Could you check a few things on this model? Use its own coordinates, in mm. A direction names the side the tool comes from. Give positions to 0.01 mm unless a question says otherwise; leave off trailing zeros. Write each loop counter-clockwise with the first axis right and the second up, starting at its lowest first coordinate (ties: lowest second). Pieces come first, ordered by that corner, then holes. Notation, with made-up numbers: (-32, 65.5) - (21, 65.5) arc R17 cw to (21, 91.5) - close; hole circle Ø6 at (29.25, 30.5). An arc over 180 degrees is marked (long way). Answer in a Markdown table with one row per item.
Autodesk Inventor part; units mm, degrees
ref_plane "YZ Plane" through (0, 0, 0) normal (1, 0, 0) x (0, 1, 0)
ref_plane "XZ Plane" through (0, 0, 0) normal (0, 1, 0) x (-1, 0, 0)
ref_plane "XY Plane" through (0, 0, 0) normal (0, 0, 1) x (1, 0, 0)
sketch "スケッチ1" plane through (0, 0, 0) normal (0, 0, 1) x (1, 0, 0)
  circle A0 centre (11, -20) radius 1.25 construction
  circle A1 centre (11, 20) radius 1.25 construction
  circle A2 centre (-11, -20) radius 1.25 construction
  arc A3 (8.5, 20) -> (11, 17.5) centre (11, 20) ccw construction
  line L0 (11, 17.5) -> (12.15, 17.5) construction
  arc A4 (13.15, 16.5) -> (12.15, 17.5) centre (12.15, 16.5) ccw construction
  line L1 (13.15, 16.5) -> (13.15, -16.5) construction
  arc A5 (12.15, -17.5) -> (13.15, -16.5) centre (12.15, -16.5) ccw construction
  line L2 (12.15, -17.5) -> (11, -17.5) construction
  arc A6 (11, -17.5) -> (8.5, -20) centre (11, -20) ccw construction
  line L3 (8.5, -20) -> (8.5, -21.15) construction
  arc A7 (7.5, -22.15) -> (8.5, -21.15) centre (7.5, -21.15) ccw construction
  line L4 (7.5, -22.15) -> (-7.5, -22.15) construction
  arc A8 (-8.5, -21.15) -> (-7.5, -22.15) centre (-7.5, -21.15) ccw construction
  line L5 (-8.5, -21.15) -> (-8.5, -20) construction
  arc A9 (-8.5, -20) -> (-11, -17.5) centre (-11, -20) ccw construction
  line L6 (-11, -17.5) -> (-14, -17.5) construction
  line L7 (8.5, 23) -> (8.5, 20) construction
  line L8 (-14.25, -17.75) -> (-14.25, -21.25) construction
  line L9 (-14.25, -21.25) -> (-12.25, -23.25)
  line L10 (-12.25, -23.25) -> (12.25, -23.25)
  line L11 (12.25, -23.25) -> (14.25, -21.25)
  line L12 (14.25, -21.25) -> (14.25, 21.25) construction
  line L13 (14.25, 21.25) -> (12.25, 23.25)
  line L14 (12.25, 23.25) -> (8.75, 23.25) construction
  line L15 (16.75, 15.618) -> (22.25, 15.618)
  line L16 (41.3, 21.118) -> (41.3, -2.882)
  line L17 (19.75, -0.382) -> (16.75, -0.382)
  arc A10 (41.3, 21.118) -> (35.8184, 22.8038) centre (38.3, 21.118) ccw
  arc A11 (39.5165, -5.6243) -> (41.3, -2.882) centre (38.3, -2.882) ccw
  circle A12 centre (38.3, 21.118) radius 1.25 construction
  circle A13 centre (38.3, -2.882) radius 1.25 construction
  line L18 (14.25, 21.25) -> (14.25, 18.118)
  line L19 (14.25, -2.882) -> (14.25, -21.25)
  arc A14 (14.25, 18.118) -> (16.75, 15.618) centre (16.75, 18.118) ccw
  arc A15 (16.75, -0.382) -> (14.25, -2.882) centre (16.75, -2.882) ccw
  line L20 (72.306, -6.882) -> (-28.676, -6.882) construction
  circle A16 centre (1.21, -13.01) radius 8.7 construction
  circle A17 centre (1.21, -13.01) radius 8.95
  arc A18 (22.25, 15.618) -> (35.8184, 22.8038) centre (22.25, 32.0211) ccw
  line L21 (22.25, 32.0211) -> (22.25, -5.382) construction
  line L22 (22.25, -2.882) -> (22.25, -5.882)
  line L23 (24.75, -8.382) -> (33.3, -8.382)
  line L24 (33.3, -8.382) -> (39.5165, -5.6243)
  arc A19 (22.25, -2.882) -> (19.75, -0.382) centre (19.75, -2.882) ccw
  arc A20 (22.25, -5.882) -> (24.75, -8.382) centre (24.75, -5.882) ccw
  circle A21 centre (0, 12) radius 1.25 construction
  line L25 (12.25, 23.25) -> (8.5, 23.25)
  line L26 (8.5, 23.25) -> (-2.0647, 20.76)
  arc A22 (-2.0647, 20.76) -> (-8.234, 15.6334) centre (0, 12) ccw
  line L27 (0, 0) -> (0, -31.805) construction
  line L28 (-12.15, -17.5) -> (-14.25, -17.5) construction
  line L29 (8.5, 23.25) -> (8.5, 21.15) construction
  line L30 (8.75, 23.25) -> (8.5, 23)
  line L31 (-14, -17.5) -> (-14.25, -17.75) construction
  line L32 (-14.25, 0) -> (-14.25, -2) construction
  line L33 (-14.25, -2) -> (-16.25, -2)
  line L34 (-16.25, -2) -> (-16.25, -5)
  line L35 (-16.25, -5) -> (-14.25, -5)
  line L36 (-14.25, -5) -> (-14.25, -7) construction
  line L37 (-14.25, 0) -> (-14.25, 2)
  line L38 (-14.25, 2) -> (-8.234, 15.6334)
  arc A23 (-14.25, -2) -> (-14.25, 0) centre (-14.25, -1) ccw
  arc A24 (-14.25, -7) -> (-14.25, -5) centre (-14.25, -6) ccw
  line L39 (-14.25, -7) -> (-14.25, -21.25)
  point P0 (11, 20)
  point P1 (11, -20)
  point P2 (-11, -20)
  point P3 (14.25, 15.618)
  point P4 (23.6679, 15.618)
  point P5 (23.161, -0.382)
  point P6 (14.25, -0.382)
  point P7 (22.25, -0.382)
  dimension "d0" = 3
  dimension "d1" = 2.5
  dimension "d2" = 6.5
  dimension "d3" = 0.25
  dimension "d7" = 16
  dimension "d8" = 8
  dimension "d16" = 8
  dimension "d17" = 5
  dimension "d26" = 9
  dimension "d34" = 1
  dimension "d35" = 3
  dimension "d36" = 2
  dimension "d37" = 10
  dimension "d38" = 2
extrude "押し出し1" add sketch "スケッチ1" along normal blind 2
sketch "スケッチ2" plane through (0, 0, 2) normal (0, 0, 1) x (1, 0, 0)
  point P0 (0, 0)
  point P1 (38.3, 21.118)
  point P2 (38.3, -2.882)
  point P3 (-11, 20)
  point P4 (11, 20)
  point P5 (11, -20)
  point P6 (-11, -20)
hole "穴2" at (38.3, 21.118, 2) at (38.3, -2.882, 2) at (-11, 20, 2) at (11, 20, 2) at (11, -20, 2) at (-11, -20, 2) direction (0, 0, -1) diameter 2.5 end through all countersink diameter 5 countersink angle 90
hole "穴3" at (0, 12, 0) direction (0, 0, 1) diameter 3 end through all
chamfer "面取り1" distance 0.25 angle 45 2 edges at (-16.25, -2, 1) (-16.25, -5, 1)
properties part number "COXA_YAW_ROLL_ADPT_TOP_BASE"
1) Imagine slicing it at A-A (y = -13.01). List the corners of the cut face in (x, z) for me.
Check values:
| item | result |
|---|---|
| outline | (-14.25, 0) - (-7.74, 0) - (-7.74, 2) - (-14.25, 2) - close; (10.16, 0) - (14.25, 0) - (14.25, 2) - (10.16, 2) - close |
2) Imagine slicing it at B-B (x = -11). List the corners of the cut face in (y, z) for me.
Check values:
| item | result |
|---|---|
| outline | (-23.25, 0) - (-21.25, 0) - (-21.25, 0.75) - (-22.5, 2) - (-23.25, 2) - close; (-18.75, 0) - (9.37, 0) - (9.37, 2) - (-17.5, 2) - (-18.75, 0.75) - close |
3) We'd pull the mould along Y, two halves only. Please class faces 1 (the face through (39.52, -2.61, 0.37)), 2 (the face through (-11.284, 8.721, 0.986)), 3 (the face through (14.25, 20, 1)): +Y half, -Y half, draft (parallel to the pull), parting line (faces both ways), or undercut.
Check values:
| item | result |
|---|---|
| face 1 | undercut |
| face 2 | +Y half |
| face 3 | draft |
4) Imagine slicing it at D-D (y = -20). List the corners of the cut face in (x, z) for me.
Check values:
| item | result |
|---|---|
| outline | (-14.25, 0) - (-12.25, 0) - (-12.25, 0.75) - (-13.5, 2) - (-14.25, 2) - close; (-9.75, 0) - (-4.38, 0) - (-4.38, 2) - (-8.5, 2) - (-9.75, 0.75) - close; (6.8, 0) - (9.75, 0) - (9.75, 0.75) - (8.5, 2) - (6.8, 2) - close; (12.25, 0) - (14.25, 0) - (14.25, 2) - (13.5, 2) - (12.25, 0.75) - close |
5) If I drill on line 1 (X direction, y = -3, z = 0.15); line 2 (X direction, y = -20, z = 0.5); line 3 (X direction, y = -13.5, z = 0.4), over which ranges is the centre line in solid material (lowest first)?
Check values:
| item | result |
|---|---|
| line 1 | x = -16.25 to 14.25, 22.25 to 37.06, 39.54 to 41.3 |
| line 2 | x = -14.25 to -12.25, -9.75 to -4.38, 6.8 to 9.75, 12.25 to 14.25 |
| line 3 | x = -14.25 to -7.73, 10.15 to 14.25 |
6) Will these pins go through, and if not, where does the flat tip stop? P1, Ø4, axis at x = 11, y = -20, coming from the +Z side; P2, Ø0.6, axis at y = -13.5, z = 1, coming from the -X side; P3, Ø1, axis at x = 29, z = 2, coming from the +Y side.
Check values:
| item | result |
|---|---|
| P1 | stops at z = 1.5 |
| P2 | stops at x = -14.25 |
| P3 | stops at y = 17.31 |
7) On a 3-axis mill with a long thin cutter (end or side, diameter ignored), from which of +Z, -Z, +X, -X, +Y, -Y can I reach the whole of each face in a straight line? I mean faces 4 (the face through (13.3, 22.2, 1)), 5 (the face through (-15, -2, 1)), 6 (the face through (23, -7.67, 0.99)). Say none if no direction works.
Check values:
| item | result |
|---|---|
| face 4 | +Z, -Z, +Y |
| face 5 | +Z, -Z, -X, +Y |
| face 6 | +Z, -Z, -Y |
8) Imagine slicing it at C-C (x = 0). List the corners of the cut face in (y, z) for me, then the cut area to 3 significant figures.
Check values:
| item | result |
|---|---|
| outline | (-23.25, 0) - (-21.88, 0) - (-21.88, 2) - (-23.25, 2) - close; (-4.14, 0) - (10.5, 0) - (10.5, 2) - (-4.14, 2) - close; (13.5, 0) - (21.25, 0) - (21.25, 2) - (13.5, 2) - close |
| area | 47.5 mm2 |
